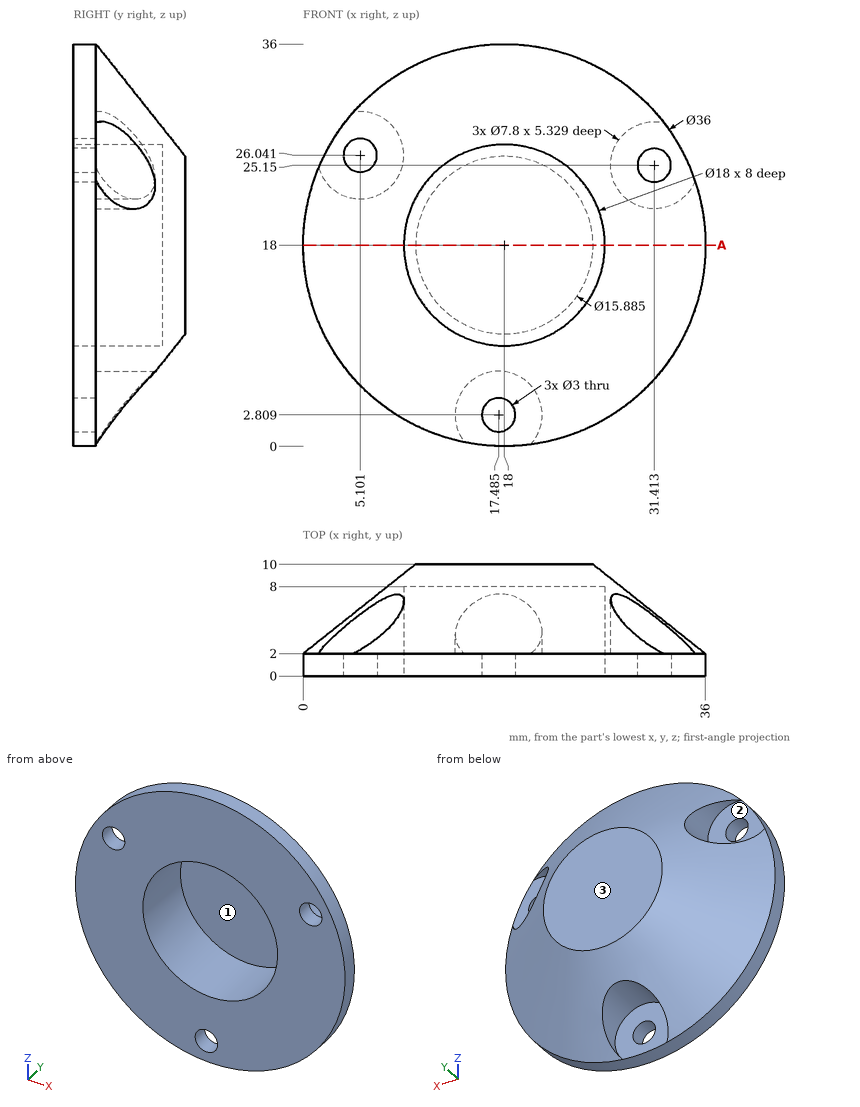
Print and shaded views of the part. All mm, measured from the part's lowest x, y and z. A direction names the side the tool comes from. Give positions to 0.01 mm unless a question says otherwise; leave off trailing zeros. Write each loop counter-clockwise with the first axis right and the second up, starting at its lowest first coordinate (ties: lowest second). Pieces come first, ordered by that corner, then holes. Notation, with made-up numbers: (-27.5, 88.25) - (7.5, 88.25) arc R8 cw to (7.5, 92.25) - close; hole circle Ø8 at (-19, 23.5). An arc over 180 degrees is marked (long way). One line per question, with ' | ' between items. Start each with the question number.
(1) 3-axis set-ups, long thin cutter, end or side, ignore diameter. For the marked faces 1, 2 and 3: which of +Z, -Z, +X, -X, +Y, -Y reach the whole face in a straight line?
(2) Wall check: line 1 along Y through (x, z) = (21.5, 12.5); line 2 along X through (y, z) = (6.5, 23.5) (1 decimal); line 3 along Z through (x, y) = (12.5, 6.25) (1 decimal). Give the ranges that are in metal, low to high. Write a range as from..to.
(3) Slice it at A-A on z = 18. Write the cut outline in (x, y).
(4) Pin check, flat tips, straight feed: P1, Ø4, axis at x = 31.5, z = 23, coming from the +Y side (1 decimal); P2, Ø1.5, axis at x = 26.5, z = 31.5, coming from the +Y side (1 decimal); P3, Ø9, axis at x = 31.41, z = 25.15, coming from the +Y side. Stop position of each tip, or through.
Results below:
1) face 1: -Y | face 2: +Y | face 3: +Z, -Z, +X, -X, +Y
2) line 1: 8..10 | line 2: 8.1..10.9, 25.1..27.9 | line 3: 6.6..10.9, 25.1..29.4
3) outline: (0, 0) - (9, 0) - (9, 8) - (27, 8) - (27, 0) - (36, 0) - (36, 2) - (25.94, 10) - (10.06, 10) - (0, 2) - close
4) P1: y = 6.2 | P2: y = 4.2 | P3: y = 7.81
